```python
from build123d import *

# Parameters (mm, degrees)
ESBO_O1_W                = 100.3
ESBO_O1_H                = 42.3
ESBO_O1_R                = 5.15
RESSALTO_EXTRUS_O1_DEPTH = 7
RESSALTO_EXTRUS_O2_START = 7
ESBO_O1_6_W              = 100.3
ESBO_O1_6_H              = 42.3
ESBO_O1_6_R              = 5.15
RESSALTO_EXTRUS_O2_DEPTH = 2
FILETE1_R                = 33
FILETE2_R                = 10


with BuildPart() as part:
    # Esboço1 → Ressalto-extrusão1 (new body)
    with BuildSketch(Plane.XY):
        with Locations((0.087398189, -10.441132561)):
            Rectangle(ESBO_O1_W, ESBO_O1_H)
        with Locations((-16.508590221, 3.558867439)):
            Circle(ESBO_O1_R, mode=Mode.SUBTRACT)
        with Locations((16.491409779, 3.558867439)):
            Circle(ESBO_O1_R, mode=Mode.SUBTRACT)
        with Locations((-39.912601811, -21.441132561)):
            Circle(ESBO_O1_R, mode=Mode.SUBTRACT)
        with Locations((40.087398189, -21.441132561)):
            Circle(ESBO_O1_R, mode=Mode.SUBTRACT)
    extrude(amount=RESSALTO_EXTRUS_O1_DEPTH)

    # Esboço1<6> → Ressalto-extrusão2 (add)
    # profile 1 of 5: a face of its own
    with BuildSketch(Plane.XY.offset(RESSALTO_EXTRUS_O2_START)):
        with Locations((0.087398189, -10.441132561)):
            Rectangle(ESBO_O1_6_W, ESBO_O1_6_H)
        with Locations((16.491409779, 3.558867439)):
            Circle(ESBO_O1_6_R, mode=Mode.SUBTRACT)
        with Locations((-16.508590221, 3.558867439)):
            Circle(ESBO_O1_6_R, mode=Mode.SUBTRACT)
        with Locations((-39.912601811, -21.441132561)):
            Circle(ESBO_O1_6_R, mode=Mode.SUBTRACT)
        with Locations((40.087398189, -21.441132561)):
            Circle(ESBO_O1_6_R, mode=Mode.SUBTRACT)
    # profile 2 of 5: a face of its own
    with BuildSketch(Plane.XY.offset(RESSALTO_EXTRUS_O2_START)):
        with Locations((40.087398189, -21.441132561)):
            Circle(ESBO_O1_6_R)
    # profile 3 of 5: a face of its own
    with BuildSketch(Plane.XY.offset(RESSALTO_EXTRUS_O2_START)):
        with Locations((-39.912601811, -21.441132561)):
            Circle(ESBO_O1_6_R)
    # profile 4 of 5: a face of its own
    with BuildSketch(Plane.XY.offset(RESSALTO_EXTRUS_O2_START)):
        with Locations((16.491409779, 3.558867439)):
            Circle(ESBO_O1_6_R)
    # profile 5 of 5: a face of its own
    with BuildSketch(Plane.XY.offset(RESSALTO_EXTRUS_O2_START)):
        with Locations((-16.508590221, 3.558867439)):
            Circle(ESBO_O1_6_R)
    extrude(amount=RESSALTO_EXTRUS_O2_DEPTH)

    # Filete1
    filete1_edges = [part.edges().sort_by_distance(p)[0] for p in [
        (50.237398189, 10.708867439, 4.5),
        (-50.062601811, 10.708867439, 4.5),
    ]]
    fillet(filete1_edges, radius=FILETE1_R)

    # Filete2
    filete2_edges = [part.edges().sort_by_distance(p)[0] for p in [
        (50.237398189, -31.591132561, 4.5),
        (-50.062601811, -31.591132561, 4.5),
    ]]
    fillet(filete2_edges, radius=FILETE2_R)


solid = part.part
```
Read the model definition and answer for the solid it produces. Units are mm, in the model's axes. A direction names the side the tool comes from. Give positions to 0.01 mm unless a question says otherwise; leave off trailing zeros. Order: outer loops, then holes, each group sorted by start corner. A loop starts at its lowest first (then second) coordinate and runs counter-clockwise, first axis right, second up.
(1) Find section C-C (z = 1). Give the number of separate pieces and of enclosed holes in the cut face, plus the area to 3 significant figures.
(2) For faces 1 (the flat face through (-1, -10, 0)), 2 (the flat face through (40, -21, 7)), determine the directions among +Z, -Z, +X, -X, +Y, -Y from which every point of the face is accessible in a straight line to the end or side of a thin tool.
(3) Find section A-A (y = 1). Give the vertices of the cut face in (x, z).
(4) For a pull along Y with two mould halves and no side action, classify faces 3 (the cylindrical face through (34.942, -21.215, 3.451)), 4 (the flat face through (-17, 4, 7)), 5 (the cylindrical face through (-40.29, 1.15, 4.44)), 6 (the flat face through (0, -31.591, 4)) as released by +Y, released by -Y, zero draft, split by the parting line, or undercut.
(5) Find section B-B (x = 36). Give the vertices of the cut face in (y, z), plus the area to 3 significant figures.
(6) Straight lines are drawn through the part: L1, parallel to X at y = -25, z = 2.5; L2, parallel to X at y = 5, z = 5.25; L3, parallel to Y at x = -19, z = 2.75. For each, find the intervals that lie inside material, in ascending order.
(7) Given pin 1 (8 mm diameter, centred on x = 17.5, y = 6, fed in from -Z); pin 2 (1 mm diameter, centred on y = -9, z = 1, fed in from +X); pin 3 (9.5 mm diameter, centred on x = -16.51, y = 3.56, fed in from -Z), each flat-ended and moving along its own axis, determine where each tip first touches the part or whether it passes through.
(8) Find section D-D (y = -19). Give the vertices of the cut face in (x, z), plus the area to 3 significant figures.
Result sheet:
1. separate pieces: 1
1. enclosed holes: 4
1. area: 3,400 mm2
2. face 1: -Z, +X, -X, +Y, -Y
2. face 2: -Z
3. outline: (-40.44, 0) - (-20.98, 0) - (-20.98, 7) - (-12.04, 7) - (-12.04, 0) - (12.02, 0) - (12.02, 7) - (20.96, 7) - (20.96, 0) - (40.62, 0) - (40.62, 9) - (-40.44, 9) - close
4. face 3: undercut
4. face 4: undercut
4. face 5: released by +Y
4. face 6: released by -Y
5. outline: (-31.59, 0) - (-24.57, 0) - (-24.57, 7) - (-18.31, 7) - (-18.31, 0) - (4.86, 0) - (4.86, 9) - (-31.59, 9) - close
5. area: 284 mm2
6. L1: x = -49.45 to -43.64, -36.19 to 36.36, 43.81 to 49.63
6. L2: x = -35.62 to -21.45, -11.56 to 11.55, 21.44 to 35.79
6. L3: y = -31.59 to -0.95, 8.07 to 10.65
7. pin 1: stops at z = 0
7. pin 2: stops at x = 47.66
7. pin 3: stops at z = 7
8. outline: (-49.9, 0) - (-44.45, 0) - (-44.45, 7) - (-35.38, 7) - (-35.38, 0) - (35.55, 0) - (35.55, 7) - (44.62, 7) - (44.62, 0) - (50.07, 0) - (50.07, 9) - (-49.9, 9) - close
8. area: 773 mm2
